from build123d import *

# Parameters (mm, degrees)
BOSS_EXTRUDE1_DEPTH         = 29
SKETCH3_W                   = 4.5
SKETCH3_H                   = 21
CUT_EXTRUDE1_DEPTH          = 6
SKETCH6_R                   = 2.15
CUT_EXTRUDE2_DEPTH          = 41.509258201
CUT_EXTRUDE3_DEPTH          = 3.5
EXTRUDE_1_REACH             = 41.674
SKETCH_1_W                  = 19.5
SKETCH_1_H                  = 14.5
EXTRUDE_1_DIRECTION_2_REACH = 41.674
SKETCH_2_W                  = 4.5
SKETCH_2_H                  = 1
CUT_EXTRUDE_1_DEPTH         = 19.5
SKETCH_4_W                  = 4
SKETCH_4_H                  = 4
CUT_EXTRUDE_3_DEPTH         = 0.7
SKETCH_5_W                  = 2
SKETCH_5_H                  = 12
CUT_EXTRUDE_4_DEPTH         = 6.25
SKETCH_6_W                  = 11
SKETCH_6_H                  = 11
CUT_EXTRUDE_5_DEPTH         = 6.25
SKETCH_7_W                  = 10.248534494
SKETCH_7_H                  = 8.686096419
CUT_EXTRUDE_6_DEPTH         = 1.75
SKETCH_8_W                  = 2
SKETCH_8_H                  = 14.5
EXTRUDE_2_DEPTH             = 10
SKETCH_9_W                  = 2
SKETCH_9_H                  = 14.5
EXTRUDE_3_DEPTH             = 7.5
FILLET_1_R                  = 1
CUT_EXTRUDE_7_DEPTH         = 41.509258201
CUT_EXTRUDE_7_DEPTH_BACK    = 41.509258201
SKETCH_10_W                 = 65.54105611
SKETCH_10_H                 = 22.030016429
CUT_EXTRUDE_8_DEPTH         = 47.588625221
CUT_EXTRUDE_8_DEPTH_BACK    = 47.588625221
SKETCH_11_W                 = 33.086172565
SKETCH_11_H                 = 28.836254029
SKETCH_12_W                 = 67
SKETCH_12_H                 = 109
EXTRUDE_4_DEPTH             = 2
EXTRUDE_3_2_DEPTH           = 25
SKETCH_13_3_W               = 33
SKETCH_13_3_H               = 2
SKETCH_13_3_W_2             = 2
SKETCH_13_3_H_2             = 94
EXTRUDE_4_2_DEPTH           = 25
EXTRUDE_5_DEPTH             = 10.5
EXTRUDE_5_2_DEPTH           = 2


with BuildPart() as part:
    # Sketch2 → Boss-Extrude1 (new body)
    with BuildSketch(Plane(origin=(0, 0, 0), x_dir=(1, 0, 0), z_dir=(0, 1, 0))):
        with BuildLine():
            Line((0, 10), (0, 20))
            Line((0, 20), (8, 20))
            Line((8, 20), (8, 14.245191882))
            ThreePointArc((8, 14.245191882), (10.672752557, 14.316274399), (13, 13))
            Line((13, 13), (9.464466094, 9.464466094))
            Line((9.464466094, 9.464466094), (2.928932188, 2.928932188))
            ThreePointArc((2.928932188, 2.928932188), (0.761204675, 6.173165676), (0, 10))
        make_face()
    boss_extrude1 = extrude(amount=BOSS_EXTRUDE1_DEPTH)

    # Mirror1: Boss-Extrude1 across plane
    add(boss_extrude1.mirror(Plane(origin=(0, 0, 0), x_dir=(-0.707106781186546, 0, 0.707106781186549), z_dir=(0.707106781186549, 0, 0.707106781186546))))

    # Sketch3 → Cut-Extrude1 (cut)
    with BuildSketch(Plane(origin=(0, 0, -20), x_dir=(-1, 0, 0), z_dir=(0, 0, -1))):
        with Locations((-4, 14.5)):
            Rectangle(SKETCH3_W, SKETCH3_H)
    cut_extrude1 = extrude(amount=-CUT_EXTRUDE1_DEPTH, mode=Mode.SUBTRACT)

    # Mirror2: Cut-Extrude1 across plane
    add(cut_extrude1.mirror(Plane(origin=(0, 0, 0), x_dir=(-0.707106781186546, 0, 0.707106781186549), z_dir=(0.707106781186549, 0, 0.707106781186546))), mode=Mode.SUBTRACT)

    # Sketch6 → Cut-Extrude2 (cut, through all)
    with BuildSketch(Plane(origin=(0, 29, 0), x_dir=(1, 0, 0), z_dir=(0, 1, 0))):
        with Locations(Location((10, 10, 0), (0, 0, 270))):
            Circle(SKETCH6_R)
    extrude(amount=-CUT_EXTRUDE2_DEPTH, mode=Mode.SUBTRACT)

    # Sketch9 → Cut-Extrude3 (cut)
    with BuildSketch(Plane(origin=(0, 24, 0), x_dir=(1, 0, 0), z_dir=(0, 1, 0))):
        Polygon((8.939052358, 13.959510504), (13.429036683, 18.44949483), (18.429313529, 13.762345089), (13.959510504, 8.939052358), (11.060947642, 6.040489496), (7.101437138, 7.101437138), (6.040489496, 11.060947642), align=None)
    cut_extrude3 = extrude(amount=-CUT_EXTRUDE3_DEPTH, mode=Mode.SUBTRACT)

    # Mirror4: Cut-Extrude3 across plane
    add(cut_extrude3.mirror(Plane.ZX.offset(14.5)), mode=Mode.SUBTRACT)


with BuildPart() as body_2:

    # Бобышка-Вытянуть1: up to this face of the body (flat: up to its plane)
    extrude_1_end = Plane(part.part.faces().sort_by_distance((17.122595941, 14.5, -8))[0])
    # Эскиз1 → Бобышка-Вытянуть1 (new, up to the picked face)
    with BuildSketch(Plane(origin=(0, 0, -1.75), x_dir=(-1, 0, 0), z_dir=(0, 0, -1)), mode=Mode.PRIVATE) as extrude_1_sk1:
        with Locations((-29.75, 7.25)):
            Rectangle(SKETCH_1_W, SKETCH_1_H)
    extrude_1_tool1 = split(extrude(extrude_1_sk1.sketch, amount=EXTRUDE_1_REACH, mode=Mode.PRIVATE), bisect_by=extrude_1_end, keep=Keep.BOTH, mode=Mode.PRIVATE)
    add(extrude_1_tool1.solids().sort_by(Axis((29.75, 7.25, -1.75), (0, 0, -1)))[0])


    # Бобышка-Вытянуть1 direction 2: up to this face of the body (flat: up to its plane)
    extrude_1_direction_2_end = Plane(part.part.faces().sort_by_distance((15, 14.5, 0))[0])
    # Эскиз1 → Бобышка-Вытянуть1 direction 2 (add, up to the picked face)
    with BuildSketch(Plane(origin=(0, 0, -1.75), x_dir=(-1, 0, 0), z_dir=(0, 0, -1)), mode=Mode.PRIVATE) as extrude_1_direction_2_sk1:
        with Locations((-29.75, 7.25)):
            Rectangle(SKETCH_1_W, SKETCH_1_H)
    extrude_1_direction_2_tool1 = split(extrude(extrude_1_direction_2_sk1.sketch, amount=-EXTRUDE_1_DIRECTION_2_REACH, mode=Mode.PRIVATE), bisect_by=extrude_1_direction_2_end, keep=Keep.BOTH, mode=Mode.PRIVATE)
    add(extrude_1_direction_2_tool1.solids().sort_by(Axis((29.75, 7.25, -1.75), (0, 0, 1)))[0])

    # Эскиз2 → Вырез-Вытянуть1 (cut)
    with BuildSketch(Plane(origin=(39.5, 0, 0), x_dir=(0, 0, -1), z_dir=(1, 0, 0))):
        with Locations((4, 14)):
            Rectangle(SKETCH_2_W, SKETCH_2_H)
    extrude(amount=-CUT_EXTRUDE_1_DEPTH, mode=Mode.SUBTRACT)

    # Эскиз4 → Вырез-Вытянуть3 (cut)
    with BuildSketch(Plane(origin=(0, 0, -8), x_dir=(-1, 0, 0), z_dir=(0, 0, -1))):
        with Locations((-22.5, 5.912430948)):
            Rectangle(SKETCH_4_W, SKETCH_4_H)
    extrude(amount=-CUT_EXTRUDE_3_DEPTH, mode=Mode.SUBTRACT)

    # Эскиз5 → Вырез-Вытянуть4 (cut)
    with BuildSketch(Plane(origin=(0, 0, -8), x_dir=(-1, 0, 0), z_dir=(0, 0, -1))):
        with Locations((-25.5, 6)):
            Rectangle(SKETCH_5_W, SKETCH_5_H)
    extrude(amount=-CUT_EXTRUDE_4_DEPTH, mode=Mode.SUBTRACT)

    # Эскиз6 → Вырез-Вытянуть5 (cut)
    with BuildSketch(Plane(origin=(0, 0, -8), x_dir=(-1, 0, 0), z_dir=(0, 0, -1))):
        with Locations((-32, 5.5)):
            Rectangle(SKETCH_6_W, SKETCH_6_H)
    extrude(amount=-CUT_EXTRUDE_5_DEPTH, mode=Mode.SUBTRACT)

    # Эскиз7 → Вырез-Вытянуть6 (cut)
    with BuildSketch(Plane(origin=(0, 0, -1.75), x_dir=(-1, 0, 0), z_dir=(0, 0, -1))):
        with Locations((-32.175732753, 6.09304821)):
            Rectangle(SKETCH_7_W, SKETCH_7_H)
    extrude(amount=-CUT_EXTRUDE_6_DEPTH, mode=Mode.SUBTRACT)

    # Эскиз8 → Бобышка-Вытянуть2 (add)
    with BuildSketch(Plane(origin=(0, 0, -8), x_dir=(-1, 0, 0), z_dir=(0, 0, -1))):
        with Locations((-38.5, 7.25)):
            Rectangle(SKETCH_8_W, SKETCH_8_H)
    extrude(amount=EXTRUDE_2_DEPTH)

    # Эскиз9 → Extrude 3 (add)
    with BuildSketch(Plane.ZY.offset(-37.5)):
        with Locations((-17, 7.25)):
            Rectangle(SKETCH_9_W, SKETCH_9_H)
    extrude(amount=EXTRUDE_3_DEPTH)

    # Скругление1
    fillet_1_edges = [body_2.edges().sort_by_distance(p)[0] for p in [
        (32.175732753, 1.75, 0),
        (27.051465506, 6.09304821, 0),
        (32.175732753, 10.436096419, 0),
        (37.3, 6.09304821, 0),
    ]]
    fillet(fillet_1_edges, radius=FILLET_1_R)

    # Эскиз12 → Extrude 4 (add)
    with BuildSketch(Plane(origin=(0, 14.5, 0), x_dir=(1, 0, 0), z_dir=(0, 1, 0))):
        with Locations((6, 54.5)):
            Rectangle(SKETCH_12_W, SKETCH_12_H)
    extrude(amount=-EXTRUDE_4_DEPTH)

    # Эскиз13 → Extrude 3 2 (add)
    with BuildSketch(Plane(origin=(0, 14.5, 0), x_dir=(1, 0, 0), z_dir=(0, 1, 0))):
        Polygon((39.5, 18), (39.5, 109), (-27.5, 109), (-27.5, 107), (37.5, 107), (37.5, 18), align=None)
    extrude(amount=-EXTRUDE_3_2_DEPTH)

    # Эскиз13<3> → Extrude 4 2 (add)
    with BuildSketch(Plane(origin=(0, 14.5, 0), x_dir=(1, 0, 0), z_dir=(0, 1, 0))):
        with Locations((4, 1)):
            Rectangle(SKETCH_13_3_W, SKETCH_13_3_H)
        with Locations((-26.5, 47)):
            Rectangle(SKETCH_13_3_W_2, SKETCH_13_3_H_2)
    extrude(amount=-EXTRUDE_4_2_DEPTH)

    # Эскиз14 → Extrude 5 (add)
    with BuildSketch(Plane.XZ):
        Polygon((20.5, 0), (39.5, 0), (39.5, -18), (37.5, -18), (37.5, -2), (20.5, -2), align=None)
    extrude(amount=EXTRUDE_5_DEPTH)

    # Эскиз15 → Extrude 5 2 (add)
    with BuildSketch(Plane.ZY.offset(27.5)):
        with BuildLine():
            Line((-94, -10.5), (-107, -10.5))
            Line((-107, -10.5), (-107, -3.5))
            ThreePointArc((-107, -3.5), (-100.5, -7.721238279), (-94, -3.5))
            Line((-94, -3.5), (-94, -10.5))
        make_face()
    extrude(amount=-EXTRUDE_5_2_DEPTH)


with BuildPart() as part_1:
    add(part.part)

    # Эскиз10 → Вырез-Вытянуть7 (cut, two sides: drawn at the far end of the back side and taken through both)
    with BuildSketch(Plane(origin=(20, 0, 0), x_dir=(0, 0, -1), z_dir=(1, 0, 0)).offset(-CUT_EXTRUDE_7_DEPTH_BACK)):
        with Locations((-4.725182995, 25.515008214)):
            Rectangle(SKETCH_10_W, SKETCH_10_H)
    extrude(amount=CUT_EXTRUDE_7_DEPTH + CUT_EXTRUDE_7_DEPTH_BACK, mode=Mode.SUBTRACT)

    # Эскиз11 → Вырез-Вытянуть8 (cut, two sides: drawn at the far end of the back side and taken through both)
    with BuildSketch(Plane(origin=(0, 14.5, 0), x_dir=(1, 0, 0), z_dir=(0, 1, 0)).offset(-CUT_EXTRUDE_8_DEPTH_BACK)):
        with Locations((3.456913717, 14.418127015)):
            Rectangle(SKETCH_11_W, SKETCH_11_H)
    extrude(amount=CUT_EXTRUDE_8_DEPTH + CUT_EXTRUDE_8_DEPTH_BACK, mode=Mode.SUBTRACT)


solid = body_2.part
Read the model definition and answer for the solid it produces. Units are mm, in the model's axes. A direction names the side the tool comes from. Coordinates: 2 decimals unless noted, no trailing zeros. Write each loop counter-clockwise with the first axis right and the second up, starting at its lowest first coordinate (ties: lowest second). Pieces come first, ordered by that corner, then holes. Notation, with made-up numbers: (61, 85.25) - (113, 85.25) arc R10 cw to (113, 102.25) - close; hole circle Ø5 at (67.5, 18). An arc over 180 degrees is marked (long way). One line per question, with ' | ' between items.
Q1. For faces 4 (the flat face through (26.7, 6, -1.75)), 5 (the flat face through (-25.5, 1, -53)), 6 (the flat face through (7, 1, -2)), 7 (the cylindrical face through (-26.51, -7.72, -100.61)), determine the directions among +Z, -Z, +X, -X, +Y, -Y from which every point of the face is accessible in a straight line to the end or side of a thin tool.
Result set:
face 4: none | face 5: +Z, -Y | face 6: -Y | face 7: -X
Q2. Find section A-A, the plane x = 32. Write down the section's boundary in (y, z), plus the area to 3 significant figures.
Result set:
outline: (-10.5, -109) - (14.5, -109) - (14.5, 0) - (11.44, 0) arc R1 ccw to (10.44, -1) - (10.44, -1.75) - (11, -1.75) - (11, -8) - (12.5, -8) - (12.5, -16) - (0, -16) - (0, -18) - (12.5, -18) - (12.5, -107) - (-10.5, -107) - close; (-10.5, -2) - (0, -2) - (0, -1.75) - (1.75, -1.75) - (1.75, -1) arc R1 ccw to (0.75, 0) - (-10.5, 0) - close | area: 326 mm^2
Q3. Find section B-B, the plane z = -75.5. Write down the section's boundary in (x, y).
Result set:
outline: (-27.5, -10.5) - (-25.5, -10.5) - (-25.5, 12.5) - (37.5, 12.5) - (37.5, -10.5) - (39.5, -10.5) - (39.5, 14.5) - (-27.5, 14.5) - close
Q4. Determine the mould class of faces 1 (the flat face through (6, 14.5, -55)), 2 (the flat face through (6, 2, 0)), 3 (the flat face through (32, 11, -5)) for opening direction Z: +Z half, -Z half, draft (parallel to the pull), parting line (faces both ways), or undercut.
Result set:
face 1: draft | face 2: +Z half | face 3: undercut
Q5. Find section C-C, the plane y = 6.75. Write down the section's boundary in (x, z), plus the area to 3 significant figures.
Result set:
outline: (-27.5, -109) - (39.5, -109) - (39.5, 0) - (38.3, 0) arc R1 ccw to (37.3, -1) - (37.3, -1.75) - (37.5, -1.75) - (37.5, -16) - (30, -16) - (30, -18) - (37.5, -18) - (37.5, -107) - (-27.5, -107) - close; (-27.5, -94) - (-25.5, -94) - (-25.5, 0) - (-27.5, 0) - close; (-12.5, -2) - (20, -2) - (20, -8) - (20.5, -8) - (20.5, -7.3) - (24.5, -7.3) - (24.5, -1.75) - (27.05, -1.75) - (27.05, -1) arc R1 ccw to (26.05, 0) - (-12.5, 0) - close | area: 654 mm^2
Q6. Find section D-D, the plane x = 14. Write down the section's boundary in (y, z), plus the area to 3 significant figures.
Result set:
outline: (-10.5, -109) - (14.5, -109) - (14.5, 0) - (-10.5, 0) - (-10.5, -2) - (12.5, -2) - (12.5, -107) - (-10.5, -107) - close | area: 310 mm^2
Q7. Consider L1, parallel to Z at x = 2, y = 6.5; L2, parallel to X at y = 5.5, z = -57; L3, parallel to Z at x = 31, y = 1.5. Determine where each line is inside the solid, lowest interval first. Write a range as [from, to].
Result set:
L1: [-109, -107], [-2, 0] | L2: [-27.5, -25.5], [37.5, 39.5] | L3: [-109, -107], [-18, -16], [-1.75, -0.34]
Q8. Each of these flat-tipped pins is pushed along its axis until it touches: P1, Ø0.8, axis at x = 22, z = -8, coming from the -Y side; P2, Ø6, axis at x = 16, z = -85, coming from the -Y side; P3, Ø4, axis at x = 32, y = 6, coming from the +Z side. Where does it stop, or does it pass through?
Result set:
P1: y = 0 | P2: y = 12.5 | P3: z = -16
